Work out the finished part from the listing and answer in its coordinate system (mm). Face numbers are marked on the shaded views. A direction names the side the tool comes from. Coordinates: 2 decimals unless noted, no trailing zeros. Order: outer loops, then holes, each group sorted by start corner. A loop starts at its lowest first (then second) coordinate and runs counter-clockwise, first axis right, second up. Notation, with made-up numbers: M 72,60 L 95,60 A34 cw 95,92 Z; hole C 81,73 d6. An arc over 180 degrees is marked long. Use a Markdown table: item, result. Add a question column.
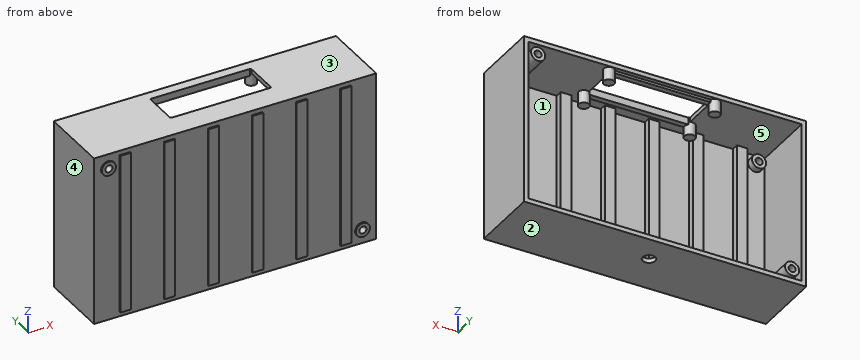
from build123d import *

# Parameters (mm, degrees)
CROQUIS1_W                   = 200
CROQUIS1_H                   = 120
SALIENTE_EXTRUIR1_DEPTH      = 50
CROQUIS2_W                   = 193.6
CROQUIS2_H                   = 113.6
CORTAR_EXTRUIR1_DEPTH        = 46
CROQUIS3_W                   = 71.5
CROQUIS3_H                   = 25.4
CORTAR_EXTRUIR2_DEPTH        = 3.5
CROQUIS4_R                   = 3.75
SALIENTE_EXTRUIR2_DEPTH      = 12.2
CROQUIS5_W                   = 71.5
CROQUIS5_H                   = 4
SALIENTE_EXTRUIR3_DEPTH      = 5
CROQUIS6_W                   = 7.5
CROQUIS6_H                   = 113.6
SALIENTE_EXTRUIR4_DEPTH      = 5
SALIENTE_EXTRUIR4_DEPTH_BACK = 5
CROQUIS7_R                   = 4.5
CORTAR_EXTRUIR3_DEPTH        = 3.3
CROQUIS6_5_R                 = 5
SALIENTE_EXTRUIR5_DEPTH      = 46
CROQUIS6_6_R                 = 5
SALIENTE_EXTRUIR6_DEPTH      = 5
SALIENTE_EXTRUIR6_DEPTH_BACK = 5
CROQUIS8_R                   = 2.5
CORTAR_EXTRUIR4_DEPTH        = 20
CROQUIS9_R                   = 2.5
CORTAR_EXTRUIR5_DEPTH        = 11


with BuildPart() as part:
    # Croquis1 → Saliente-Extruir1 (new body)
    with BuildSketch(Plane(origin=(0, 0, 0), x_dir=(1, 0, 0), z_dir=(0, 1, 0))):
        Rectangle(CROQUIS1_W, CROQUIS1_H)
    extrude(amount=SALIENTE_EXTRUIR1_DEPTH)

    # Croquis2 → Cortar-Extruir1 (cut)
    with BuildSketch(Plane(origin=(0, 50, 0), x_dir=(1, 0, 0), z_dir=(0, 1, 0))):
        Rectangle(CROQUIS2_W, CROQUIS2_H)
    extrude(amount=-CORTAR_EXTRUIR1_DEPTH, mode=Mode.SUBTRACT)

    # Croquis3 → Cortar-Extruir2 (cut)
    with BuildSketch(Plane.XY.offset(60)):
        with Locations((0, 30.3)):
            Rectangle(CROQUIS3_W, CROQUIS3_H)
    extrude(amount=-CORTAR_EXTRUIR2_DEPTH, mode=Mode.SUBTRACT)

    # Croquis4 → Saliente-Extruir2 (add)
    with BuildSketch(Plane.XY.offset(60)):
        with Locations((-37.5, 45.8)):
            Circle(CROQUIS4_R)
        with Locations((37.5, 45.8)):
            Circle(CROQUIS4_R)
        with Locations((37.5, 14.8)):
            Circle(CROQUIS4_R)
        with Locations((-37.5, 14.8)):
            Circle(CROQUIS4_R)
    extrude(amount=-SALIENTE_EXTRUIR2_DEPTH)

    # Croquis5 → Saliente-Extruir3 (add)
    with BuildSketch(Plane.XY.offset(60)):
        with Locations((0, 15.6)):
            Rectangle(CROQUIS5_W, CROQUIS5_H)
        with Locations((0, 45)):
            Rectangle(CROQUIS5_W, CROQUIS5_H)
    extrude(amount=-SALIENTE_EXTRUIR3_DEPTH)

    # Croquis6 → Saliente-Extruir4 (add, two sides)
    with BuildSketch(Plane(origin=(0, 4, 0), x_dir=(1, 0, 0), z_dir=(0, 1, 0))) as saliente_extruir4_sk:
        with Locations((-78.05, 0)):
            Rectangle(CROQUIS6_W, CROQUIS6_H)
        with Locations((-46.83, 0)):
            Rectangle(CROQUIS6_W, CROQUIS6_H)
        with Locations((-15.61, 0)):
            Rectangle(CROQUIS6_W, CROQUIS6_H)
        with Locations((15.61, 0)):
            Rectangle(CROQUIS6_W, CROQUIS6_H)
        with Locations((46.83, 0)):
            Rectangle(CROQUIS6_W, CROQUIS6_H)
        with Locations((78.05, 0)):
            Rectangle(CROQUIS6_W, CROQUIS6_H)
    extrude(amount=SALIENTE_EXTRUIR4_DEPTH)
    extrude(saliente_extruir4_sk.sketch, amount=-SALIENTE_EXTRUIR4_DEPTH_BACK)

    # Croquis7 → Cortar-Extruir3 (cut)
    with BuildSketch(Plane(origin=(0, 0, -60), x_dir=(-1, 0, 0), z_dir=(0, 0, -1))):
        with Locations((0, 30)):
            Circle(CROQUIS7_R)
    extrude(amount=-CORTAR_EXTRUIR3_DEPTH, mode=Mode.SUBTRACT)

    # Croquis6_5 → Saliente-Extruir5 (add)
    with BuildSketch(Plane(origin=(0, 4, 0), x_dir=(1, 0, 0), z_dir=(0, 1, 0))):
        with Locations((-90, 50)):
            Circle(CROQUIS6_5_R)
        with Locations((90, -50)):
            Circle(CROQUIS6_5_R)
    extrude(amount=SALIENTE_EXTRUIR5_DEPTH)

    # Croquis6_6 → Saliente-Extruir6 (add, two sides)
    with BuildSketch(Plane(origin=(0, 4, 0), x_dir=(1, 0, 0), z_dir=(0, 1, 0))) as saliente_extruir6_sk:
        with Locations((90, 50)):
            Circle(CROQUIS6_6_R)
        with Locations((-90, -50)):
            Circle(CROQUIS6_6_R)
    extrude(amount=SALIENTE_EXTRUIR6_DEPTH)
    extrude(saliente_extruir6_sk.sketch, amount=-SALIENTE_EXTRUIR6_DEPTH_BACK)

    # Croquis8 → Cortar-Extruir4 (cut)
    with BuildSketch(Plane(origin=(0, 50, 0), x_dir=(1, 0, 0), z_dir=(0, 1, 0))):
        with Locations((-90, 50)):
            Circle(CROQUIS8_R)
        with Locations((90, -50)):
            Circle(CROQUIS8_R)
    extrude(amount=-CORTAR_EXTRUIR4_DEPTH, mode=Mode.SUBTRACT)

    # Croquis9 → Cortar-Extruir5 (cut, through all)
    with BuildSketch(Plane(origin=(0, 9, 0), x_dir=(1, 0, 0), z_dir=(0, 1, 0))):
        with Locations((-90, -50)):
            Circle(CROQUIS9_R)
        with Locations((90, 50)):
            Circle(CROQUIS9_R)
    extrude(amount=-CORTAR_EXTRUIR5_DEPTH, mode=Mode.SUBTRACT)


solid = part.part
(1) A cutting plane is placed at B-B on x = 90. Write down the section's boundary in (y, z), plus the area to 3 significant figures.
(2) A cutting plane is placed at D-D on z = 50. Count the separate pieces of the cut face and the enclosed holes in it, plus the area to 3 significant figures.
(3) Straight lines are drawn through the part: line 1 (Z direction, x = -90, y = 41); line 2 (X direction, y = 41.25, z = -50); line 3 (Z direction, x = -75, y = 36.5). For each, find the intervals that lie inside material, in ascending order.
(4) Which of the six approach directions +Z, -Z, +X, -X, +Y, -Y give full straight-line access (tool end or side, diameter ignored) to the marked faces 1 and 2?
(5) Given P1, Ø0.5, axis at x = -47.5, y = -0.5, coming from the +Z side; P2, Ø1.5, axis at x = 3.5, y = 27.5, coming from the +Z side; P3, Ø3, axis at x = -36, z = -16.5, coming from the -Y side, each flat-ended and moving along its own axis, determine where each tip first touches the part or whether it passes through.
(6) The mould has two halves that part along X. Classify the marked faces 3, 4 and 5: pulls with the +X half, pulls with the -X half, needs draft (parallel to the pull), parting line crosses it, or undercut.
(7) A cutting plane is placed at A-A on x = 0. Write down the section's boundary in (y, z).
(8) A cutting plane is placed at C-C on x = 59.5. Write down the section's boundary in (y, z).
From the geometry:
| question | item | result |
|---|---|---|
| 1 | outline | M -1,-55 L 0,-55 L 0,-60 L 50,-60 L 50,-56.8 L 4,-56.8 L 4,-55 L 9,-55 L 9,-52.5 L -1,-52.5 Z; M -1,-47.5 L 9,-47.5 L 9,-45 L 4,-45 L 4,45 L 50,45 L 50,47.5 L 30,47.5 L 30,52.5 L 50,52.5 L 50,55 L 4,55 L 4,56.8 L 50,56.8 L 50,60 L 0,60 L 0,-45 L -1,-45 Z |
| 1 | area | 1,140 mm2 |
| 2 | separate pieces | 6 |
| 2 | enclosed holes | 0 |
| 2 | area | 1,910 mm2 |
| 3 | line 1 | z = -60 to -56.8, -55 to -52.5, -47.5 to -45, 56.8 to 60 |
| 3 | line 2 | x = -100 to -96.8, -95 to -92.5, -87.5 to -85, 96.8 to 100 |
| 3 | line 3 | z = -60 to -56.8, 56.8 to 60 |
| 4 | face 1 | +Y |
| 4 | face 2 | -Z, +X, -X, +Y, -Y |
| 5 | P1 | stops at z = 56.8 |
| 5 | P2 | stops at z = -56.8 |
| 5 | P3 | stops at y = 0 |
| 6 | face 3 | needs draft |
| 6 | face 4 | pulls with the -X half |
| 6 | face 5 | undercut |
| 7 | outline | M 0,-60 L 25.5,-60 L 25.5,-56.8 L 4,-56.8 L 4,56.8 L 13.6,56.8 L 13.6,55 L 17.6,55 L 17.6,60 L 0,60 Z; M 34.5,-60 L 50,-60 L 50,-56.8 L 34.5,-56.8 Z; M 43,55 L 47,55 L 47,56.8 L 50,56.8 L 50,60 L 43,60 Z |
| 8 | outline | M 0,-60 L 50,-60 L 50,-56.8 L 4,-56.8 L 4,56.8 L 50,56.8 L 50,60 L 0,60 Z |
